```python
from build123d import *

# Parameters (mm, degrees)
F0_R     = 25
F0_R_2   = 1.6
F1_DEPTH = 5
F2_R     = 12.5
F3_DEPTH = 51.2


with BuildPart() as f1:
    # F0 (on Front) → F1 (new body)
    with BuildSketch(Plane.XZ):
        Circle(F0_R)
        with Locations((-14.142136, -14.142136)):
            Circle(F0_R_2, mode=Mode.SUBTRACT)
        with Locations((14.142136, -14.142136)):
            Circle(F0_R_2, mode=Mode.SUBTRACT)
        with Locations((-14.142136, 14.142136)):
            Circle(F0_R_2, mode=Mode.SUBTRACT)
        with Locations((14.142136, 14.142136)):
            Circle(F0_R_2, mode=Mode.SUBTRACT)
    extrude(amount=F1_DEPTH)

    # F2 (on face) → F3 (cut)
    with BuildSketch(Plane.XZ.offset(5)):
        Circle(F2_R)
    extrude(amount=-F3_DEPTH, mode=Mode.SUBTRACT)


solid = f1.part
```
CAD build for the part. Positions are in the model's coordinates, mm. Round coordinates to 2 decimals unless told otherwise and drop trailing zeros. Order: outer loops, then holes, each group sorted by start corner. A loop starts at its lowest first (then second) coordinate and runs counter-clockwise, first axis right, second up. Notation, with made-up numbers: (87.5, 89.5) - (134.5, 89.5) arc R10 ccw to (134.5, 93.5) - close; hole circle Ø11 at (-26.75, 15). An arc over 180 degrees is marked (long way). Use CSV: the item, a comma, the result in double quotes. Start each with the question number.
1) Saw through at B-B (z = 0). List the corners of the cut face in (x, y), and give its area (3 significant figures).
2) Saw through at D-D (z = 13.5). List the corners of the cut face in (x, y).
3) Pin check, flat tips, straight feed: pin 1 Ø1 at (y, z) = (-3, 10) entering from +X; pin 2 Ø1 at (y, z) = (-4, 16) entering from -X; pin 3 Ø1.9 at (x, z) = (-14.14, -14.14) entering from +Y. Stop position of each tip, or through.
4) Saw through at C-C (y = -2.8). List the corners of the cut face in (x, z).
5) Two-plate mould, pull along X, no slides. Class faces 1 (the cylindrical face through (13.8, -2.46, 12.58)), 2 (the flat face through (-11.5, -5, 5.9)), 3 (the cylindrical face through (23.846, -2.465, 7.509)): pulls with the +X half, pulls with the -X half, needs draft (parallel to the pull), parting line crosses it, or undercut.
6) Wall check: L1, parallel to X at y = -0.7, z = -14; L2, parallel to Z at x = -2, y = -2.95; L3, parallel to Z at x = -8, y = -4.5. Give the ranges that are in metal, low to high. Write a range as [from, to].
7) Saw through at A-A (x = 0). List the corners of the cut face in (y, z).
Values follow:
1,outline,"(-25, -5) - (-12.5, -5) - (-12.5, 0) - (-25, 0) - close; (12.5, -5) - (25, -5) - (25, 0) - (12.5, 0) - close"
1,area,"125 mm2"
2,outline,"(-21.04, -5) - (-15.61, -5) - (-15.61, 0) - (-21.04, 0) - close; (-12.68, -5) - (12.68, -5) - (12.68, 0) - (-12.68, 0) - close; (15.61, -5) - (21.04, -5) - (21.04, 0) - (15.61, 0) - close"
3,pin 1,"stops at x = 23.12"
3,pin 2,"stops at x = -19.62"
3,pin 3,"passes through"
4,outline,"circle Ø50 at (0, 0); hole circle Ø3.2 at (-14.14, -14.14); hole circle Ø3.2 at (-14.14, 14.14); hole circle Ø25 at (0, 0); hole circle Ø3.2 at (14.14, -14.14); hole circle Ø3.2 at (14.14, 14.14)"
5,face 1,"undercut"
5,face 2,"needs draft"
5,face 3,"parting line crosses it"
6,L1,"x = [-20.71, -15.74], [-12.55, 12.55], [15.74, 20.71]"
6,L2,"z = [-24.92, -12.34], [12.34, 24.92]"
6,L3,"z = [-23.69, -9.6], [9.6, 23.69]"
7,outline,"(-5, -25) - (0, -25) - (0, -12.5) - (-5, -12.5) - close; (-5, 12.5) - (0, 12.5) - (0, 25) - (-5, 25) - close"
